Work out the finished part from the listing and answer in its coordinate system (mm). A direction names the side the tool comes from. Give positions to 0.01 mm unless a question says otherwise; leave off trailing zeros. Write each loop counter-clockwise with the first axis right and the second up, starting at its lowest first coordinate (ties: lowest second). Pieces come first, ordered by that corner, then holes. Notation, with made-up numbers: (38, -2.75) - (49, -2.75) arc R26 ccw to (49, 15.25) - close; hole circle Ø10 at (53.5, 79). An arc over 180 degrees is marked (long way). Write item = value, one per line.
from build123d import *

# Parameters (mm, degrees)
F1_DEPTH  = 17.5
F2_W      = 16.5
F2_H      = 20
F3_DEPTH  = 11
F4_R      = 1.75
F6_DEPTH  = 22.5
F8_DEPTH  = 7.5
F9_DEPTH  = 13.1
F10_DEPTH = 24.9
F11_R     = 1.75
F12_DEPTH = 2
F13_W     = 15.5
F13_H     = 6.6
F13_H_2   = 5.4
F14_DEPTH = 25
F15_DEPTH = 16.5
F17_DEPTH = 25
F18_W     = 1.5
F18_H     = 3
F19_DEPTH = 25
F21_DEPTH = 15.5
F22_SIZE  = 1.99999
F23_SIZE  = 2


# Not quite as in the source:
# - a fillet or chamfer is up to 0.001 mm smaller than in the source, because OpenCascade refuses the exact size


with BuildPart() as f1:
    # F0 (on Front) → F1 (new body)
    with BuildSketch(Plane.XZ):
        with BuildLine():
            Line((16.5, 21), (16.5, 21.3678174192))
            Line((16.5, 21.3678174192), (16.5, 38.5))
            Line((16.5, 38.5), (11.9580992435, 38.5))
            ThreePointArc((11.9580992435, 38.5), (11.8488094961, 35.2539844758), (9.3668783978, 33.1590909091))
            ThreePointArc((9.3668783978, 33.1590909091), (8.25, 29.3900555271), (7.1331216022, 33.1590909091))
            ThreePointArc((7.1331216022, 33.1590909091), (4.6511905039, 35.2539844758), (4.5419007565, 38.5))
            Line((4.5419007565, 38.5), (0, 38.5))
            Line((0, 38.5), (0, 21.3678174192))
            Line((0, 21.3678174192), (0, 21))
            Line((0, 21), (8.25, 21))
            Line((8.25, 21), (16.5, 21))
        make_face()
    extrude(amount=F1_DEPTH)

    # F2 (on face) → F3 (join)
    with BuildSketch(Plane(origin=(0, 0, 0), x_dir=(-1, 0, 0), z_dir=(0, 1, 0))):
        with Locations((-8.25, 11)):
            Rectangle(F2_W, F2_H)
    extrude(amount=-F3_DEPTH)

    # F4 (on face) → F6 (cut)
    with BuildSketch(Plane(origin=(0, 0, 0), x_dir=(-1, 0, 0), z_dir=(0, 1, 0))):
        with Locations((-11.5, 19.5)):
            Circle(F4_R)
    extrude(amount=-F6_DEPTH, mode=Mode.SUBTRACT)

    # F7 (on face) → F8 (cut)
    with BuildSketch(Plane.XZ.offset(11)):
        Polygon((14.1428062528, 17.6374994111), (14.4343759509, 20.8574870578), (11.7915696981, 22.7199876466), (8.8571937472, 21.3625005889), (8.5656240491, 18.1425129422), (11.2084303019, 16.2800123534), align=None)
    extrude(amount=-F8_DEPTH, mode=Mode.SUBTRACT)

    # F7 (on face) → F9 (cut)
    with BuildSketch(Plane.XZ.offset(11)):
        Polygon((14.1428062528, 17.6374994111), (14.4343759509, 20.8574870578), (11.7915696981, 22.7199876466), (8.8571937472, 21.3625005889), (8.5656240491, 18.1425129422), (11.2084303019, 16.2800123534), align=None)
    extrude(amount=F9_DEPTH, mode=Mode.SUBTRACT)

    # F5 (on face) → F10 (cut)
    with BuildSketch(Plane(origin=(0, 0, 0), x_dir=(0, -1, 0), z_dir=(-1, 0, 0))):
        with BuildLine():
            Line((11, 16.5), (11, 21))
            ThreePointArc((11, 21), (6.5, 16.5), (11, 12))
            Line((11, 12), (11, 16.5))
        make_face()
    extrude(amount=-F10_DEPTH, mode=Mode.SUBTRACT)

    # F11 (on face) → F12 (cut)
    with BuildSketch(Plane(origin=(0, 0, 0), x_dir=(-1, 0, 0), z_dir=(0, 1, 0))):
        with BuildLine():
            Line((-11.9580992435, 38.5), (-16.5, 38.5))
            Line((-16.5, 38.5), (-16.5, 1))
            Line((-16.5, 1), (0, 1))
            Line((0, 1), (0, 38.5))
            Line((0, 38.5), (-4.5419007565, 38.5))
            ThreePointArc((-4.5419007565, 38.5), (-4.6511905039, 35.2539844758), (-7.1331216022, 33.1590909091))
            ThreePointArc((-7.1331216022, 33.1590909091), (-8.25, 29.3900555271), (-9.3668783978, 33.1590909091))
            ThreePointArc((-9.3668783978, 33.1590909091), (-11.8488094961, 35.2539844758), (-11.9580992435, 38.5))
        make_face()
        with Locations((-11.5, 19.5)):
            Circle(F11_R, mode=Mode.SUBTRACT)
    extrude(amount=-F12_DEPTH, mode=Mode.SUBTRACT)

    # F13 (on face) → F14 (join)
    with BuildSketch(Plane.YZ.offset(16.5)):
        with Locations((-9.75, 41.8)):
            Rectangle(F13_W, F13_H)
        with Locations((-9.75, 35.8)):
            Rectangle(F13_W, F13_H_2)
    extrude(amount=F14_DEPTH)

    # F15 (add): a face of the model
    f15_faces = [f1.faces().sort_by_distance(p)[0] for p in [
        (16.5, -9.75, 41.8),
    ]]
    extrude(f15_faces, amount=F15_DEPTH)

    # F16 (on face) → F17 (cut)
    with BuildSketch(Plane(origin=(0, -2, 0), x_dir=(-1, 0, 0), z_dir=(0, 1, 0))):
        with BuildLine():
            ThreePointArc((-30.0731763785, 39.739389973), (-29, 35.9427381873), (-27.9268236215, 39.739389973))
            ThreePointArc((-27.9268236215, 39.739389973), (-25.4094368312, 41.8298269216), (-25.2948465851, 45.1))
            Line((-25.2948465851, 45.1), (-32.7051534149, 45.1))
            ThreePointArc((-32.7051534149, 45.1), (-32.5905631688, 41.8298269216), (-30.0731763785, 39.739389973))
        make_face()
    extrude(amount=-F17_DEPTH, mode=Mode.SUBTRACT)

    # F18 (on face) → F19 (cut)
    with BuildSketch(Plane.XY.offset(45.1)):
        with Locations((21.5448465851, -14)):
            Rectangle(F18_W, F18_H)
        with Locations((36.4551534149, -14)):
            Rectangle(F18_W, F18_H)
    extrude(amount=-F19_DEPTH, mode=Mode.SUBTRACT)

    # F20 (on face) → F21 (join)
    with BuildSketch(Plane.XZ.offset(17.5)):
        with BuildLine():
            Line((10.089985095, 38.5), (10.0875691268, 38.5))
            Line((10.0875691268, 38.5), (4.5419007565, 38.5))
            ThreePointArc((4.5419007565, 38.5), (4.6511905039, 35.2539844758), (7.1331216022, 33.1590909091))
            ThreePointArc((7.1331216022, 33.1590909091), (8.25, 29.3900555271), (9.3668783978, 33.1590909091))
            ThreePointArc((9.3668783978, 33.1590909091), (11.8488094961, 35.2539844758), (11.9580992435, 38.5))
            Line((11.9580992435, 38.5), (10.089985095, 38.5))
        make_face()
    extrude(amount=-F21_DEPTH)

    # F22 (size 2 in the source; OpenCascade refuses exactly that, so slightly less here)
    f22_edges = [f1.edges().sort_by_distance(p)[0] for p in [
        (41.5, -17.5, 39.1),
        (0, -17.5, 33.05),
        (16.5, -17.5, 27.05),
        (29, -17.5, 33.1),
        (12.647423, -17.5, 45.1),
        (37.102577, -17.5, 45.1),
    ]]
    chamfer(f22_edges, length=F22_SIZE)

    # F23
    f23_edges = [f1.edges().sort_by_distance(p)[0] for p in [
        (0, -11, 6.5),
        (16.5, -11, 6.5),
    ]]
    chamfer(f23_edges, length=F23_SIZE)


solid = f1.part
1. Find section B-B, the plane z = 19.5. Give the vertices of the cut face in (x, y), then the cut area to 3 significant figures.
Solution:
outline = (0, -7.65) - (8.69, -7.65) - (8.69, -3.5) - (9.75, -3.5) - (9.75, -2) - (0, -2) - close; (13.25, -3.5) - (14.31, -3.5) - (14.31, -7.65) - (16.5, -7.65) - (16.5, -2) - (13.25, -2) - close
area = 64.6 mm^2
2. For a pull along Y with two mould halves and no side action, classify faces 1 (the cylindrical face through (32.61, -9.64, 41.87)), 2 (the flat face through (8, -11, 7)), 3 (the flat face through (36, -15.5, 39)) as pulls with the +Y half, pulls with the -Y half, needs draft (parallel to the pull), parting line crosses it, or undercut.
Solution:
face_1 = needs draft
face_2 = pulls with the -Y half
face_3 = undercut
3. Straight lines are drawn through the part: line 1 (X direction, y = -12.75, z = 41.5); line 2 (Z direction, x = 11.5, y = -2.9); line 3 (Y direction, x = 21, z = 36.5). For each, find the intervals that lie inside material, in ascending order.
Solution:
line_1 = 0 to 20.79, 22.29 to 25.59, 32.41 to 35.71, 37.21 to 41.5
line_2 = 1 to 17.75, 21.25 to 45.1
line_3 = -17.5 to -15.5, -12.5 to -2
4. Given pin 1 (2 mm diameter, centred on x = 3, y = -14, fed in from -Z); pin 2 (3 mm diameter, centred on x = 12.5, z = 19, fed in from -Y); pin 3 (5.5 mm diameter, centred on x = 11.5, z = 9, fed in from -Y), each flat-ended and moving along its own axis, determine where each tip first touches the part or whether it passes through.
Solution:
pin_1 = 21
pin_2 = -3.5
pin_3 = -11
5. Find section D-D, the plane x = 34.5. Give the vertices of the cut face in (y, z).
Solution:
outline = (-17.5, 35.1) - (-15.5, 33.1) - (-2, 33.1) - (-2, 45.1) - (-15.5, 45.1) - (-17.5, 43.1) - close
6. A tool of negligible diameter and unlimited length cuts with its end or side. For faces 4 (the flat face through (10.34, -10.4, 22.05)), 5 (the flat face through (16.5, -7, 20)), 6 (the flat face through (22.295, -14, 39)), 7 (the flat face through (1, -10, 7)), 8 (the flat face through (4, -14, 21)), from which of +Z, -Z, +X, -X, +Y, -Y can it reach the whole face along a straight path? Write none if from no direction.
Solution:
face_4 = -Y
face_5 = -Z, +X, +Y, -Y
face_6 = +Z, -Z
face_7 = -Z, -X, -Y
face_8 = -Z, +X, -X, -Y
7. Find section A-A, the plane y = -14. Give the vertices of the cut face in (x, z).
Solution:
outline = (0, 21) - (8.82, 21) - (8.86, 21.36) - (11.79, 22.72) - (14.23, 21) - (16.5, 21) - (16.5, 33.1) - (20.79, 33.1) - (20.79, 45.1) - (0, 45.1) - close; (22.29, 33.1) - (35.71, 33.1) - (35.71, 45.1) - (32.71, 45.1) arc R4 cw to (30.07, 39.74) arc R2.05 cw (long way) to (27.93, 39.74) arc R4 cw to (25.29, 45.1) - (22.29, 45.1) - close; (37.21, 33.1) - (41.5, 33.1) - (41.5, 45.1) - (37.21, 45.1) - close
8. Find section C-C, the plane y = -7.5. Give the vertices of the cut face in (x, z), then the cut area to 3 significant figures.
Solution:
outline = (0, 1) - (16.5, 1) - (16.5, 13.67) - (0, 13.67) - close; (0, 19.33) - (8.67, 19.33) - (8.86, 21.36) - (11.79, 22.72) - (14.43, 20.86) - (14.3, 19.33) - (16.5, 19.33) - (16.5, 33.1) - (41.5, 33.1) - (41.5, 45.1) - (32.71, 45.1) arc R4 cw to (30.07, 39.74) arc R2.05 cw (long way) to (27.93, 39.74) arc R4 cw to (25.29, 45.1) - (0, 45.1) - close
area = 870 mm^2
